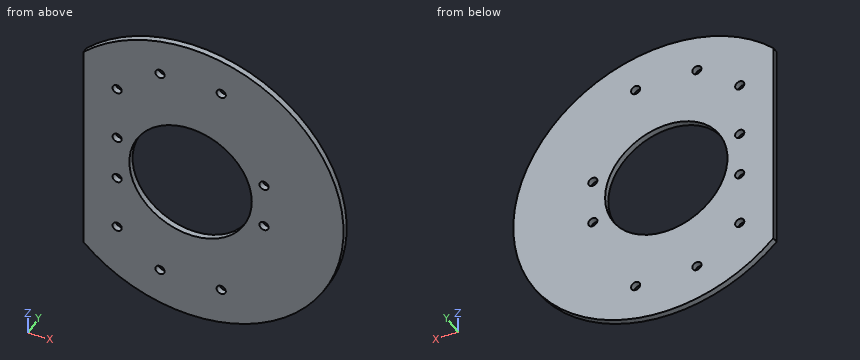
```python
from build123d import *

# Parameters (mm, degrees)
SKETCH1_R           = 20
BOSS_EXTRUDE1_DEPTH = 2
SKETCH2_R           = 1.5
SKETCH2_R_2         = 1
CUT_EXTRUDE1_DEPTH  = 2


with BuildPart() as part:
    # Sketch1 → Boss-Extrude1 (new body)
    with BuildSketch(Plane(origin=(0, 0, 0), x_dir=(1, 0, 0), z_dir=(0, 1, 0))):
        with BuildLine():
            Line((-35, 35.707142143), (-35, -35.707142143))
            ThreePointArc((-35, -35.707142143), (50, 0), (-35, 35.707142143))
        make_face()
        Circle(SKETCH1_R, mode=Mode.SUBTRACT)
    extrude(amount=BOSS_EXTRUDE1_DEPTH)

    # Sketch2 → Cut-Extrude1 (cut)
    with BuildSketch(Plane(origin=(0, 2, 0), x_dir=(1, 0, 0), z_dir=(0, 1, 0))):
        with Locations((-23.99076058, 7.565582695)):
            Circle(SKETCH2_R)
        with Locations((24.00923942, 7.565582695)):
            Circle(SKETCH2_R)
        with Locations((-23.99076058, -25.834417305)):
            Circle(SKETCH2_R)
        with Locations((-9.99076058, -36.834417305)):
            Circle(SKETCH2_R)
        with Locations((10.00923942, -36.834417305)):
            Circle(SKETCH2_R)
        with Locations((0.00923942, 0.065582695)):
            Circle(SKETCH2_R_2)
    cut_extrude1 = extrude(amount=-CUT_EXTRUDE1_DEPTH, mode=Mode.SUBTRACT)

    # Mirror1: Cut-Extrude1 across plane
    add(cut_extrude1.mirror(Plane.XY), mode=Mode.SUBTRACT)


solid = part.part
```
Can you work these out from the model? Positions are in its coordinate system, mm. Give positions to 0.01 mm unless a question says otherwise; leave off trailing zeros. Loops run counter-clockwise (first coordinate to the right, second up) from the corner with the lowest first, then second, coordinate; pieces in that order, holes last. Notation, with made-up numbers: M 55.25,8.25 L 73.25,8.25 A24 ccw 73.25,42.25 Z; hole C 79.25,58.5 d2. An arc over 180 degrees is marked long. One line per item, written item: value.
(1) Suppose I cut it at A-A on x = 0. List the corners of the cut face in (y, z) for me.
Returned:
outline: M 0,-50 L 2,-50 L 2,-20 L 0,-20 Z; M 0,20 L 2,20 L 2,50 L 0,50 Z
(2) Suppose I cut it at D-D on x = -30. List the corners of the cut face in (y, z) for me, plus the area to 3 significant figures.
Returned:
outline: M 0,-40 L 2,-40 L 2,40 L 0,40 Z
area: 160 mm^2
(3) Suppose I cut it at C-C on y = 0.8. Count the separate pieces of the cut face and the enclosed holes in it, plus the area to 3 significant figures.
Returned:
separate pieces: 1
enclosed holes: 11
area: 5,790 mm^2
(4) Suppose I cut it at B-B on z = 0. List the corners of the cut face in (x, y) for me.
Returned:
outline: M -35,0 L -20,0 L -20,2 L -35,2 Z; M 20,0 L 50,0 L 50,2 L 20,2 Z
(5) I need wall thicknesses on line 1 (X direction, y = 0.6, z = -1); line 2 (X direction, y = 1.1, z = -7) (3 decimals); line 3 (X direction, y = 0.3, z = 7.5). Which ranges of each line are inside material? Lowest first, please.
Returned:
line 1: -35 to -19.97, 19.97 to 49.99
line 2: -35 to -25.38, -22.601 to -18.735, 18.735 to 22.62, 25.399 to 49.508
line 3: -35 to -25.49, -22.49 to -18.54, 18.54 to 22.51, 25.51 to 49.43
(6) Will these pins go through, and if not, where does the flat tip stop? pin 1 (1.8 mm diameter, centred on x = -23.99, z = -25.83, fed in from +Y); pin 2 (1 mm diameter, centred on y = 0.5, z = -25.5, fed in from +X).
Returned:
pin 1: through
pin 2: x = 43.3
